The listing builds one solid part. Answer for the finished solid, in the listing's coordinates (mm). A direction names the side the tool comes from. Round coordinates to 2 decimals unless told otherwise and drop trailing zeros. Loops run counter-clockwise (first coordinate to the right, second up) from the corner with the lowest first, then second, coordinate; pieces in that order, holes last. Notation, with made-up numbers: (-12, 72.5) -> (-5, 72.5) arc R19 cw to (-5, 107.5) -> close; hole circle Ø11 at (22.5, -25.75). An arc over 180 degrees is marked (long way). Write each question's results on one line, items separated by ' | '. Start each with the question number.
(1) The part is cut by section B-B (y = 4). Determine the outline of the cut face in (x, z).
(2) The part is cut by section C-C (x = -8.5). Determine the outline of the cut face in (y, z).
(3) Flat-ended cylindrical pins translate along their axes: pin 1 (5 mm diameter, centred on y = 18.5, z = 7.5, fed in from -X); pin 2 (3 mm diameter, centred on y = 26, z = 6.5, fed in from -X); pin 3 (5.5 mm diameter, centred on x = 0, z = 0, fed in from -Y); pin 4 (6 mm diameter, centred on x = -6.5, z = -4, fed in from +Y). Find the tip coordinate at first contact, or state that the pin passes through.
(4) For faces 1 (the face through (-5, 22, 2)), 2 (the face through (0, 37, 0)), 3 (the face through (2.86, 7.89, 0.9)), 4 (the face through (0.62, 2.8, -6.29)), determine the directions among +Z, -Z, +X, -X, +Y, -Y from which every point of the face is accessible in a straight line to the end or side of a thin tool.
(5) The part is cut by section A-A (z = 0). Determine the outline of the cut face in (x, y).
(6) Determine the mould class of faces 5 (the face through (2.1, 0, -2.4)), 6 (the face through (0, 16, 0)), 7 (the face through (-6.29, 2.8, -0.62)), 8 (the face through (9.237, 10.846, 3.83)) for opening direction Z: released by +Z, released by -Z, zero draft, split by the parting line, or undercut.
(7) The part is cut by section D-D (z = -7.25). Determine the outline of the cut face in (x, y), plus the area to 3 significant figures.
(8) Straight lines are drawn through the part: probe 1 along Y at (x, z) = (0, -7); probe 2 along Y at (x, z) = (2.25, 5.5); probe 3 along Z at (x, y) = (-4.5, 4). For each, find the intervals that lie inside material, in ascending order.
```python
from build123d import *

# Parameters (mm, degrees)
SKETCH_1_R          = 10
EXTRUDE_1_DEPTH     = 22
SKETCH_2_R          = 4
EXTRUDE_2_DEPTH     = 15
FILLET_1_R          = 1
CHAMFER_1_SIZE      = 1
SKETCH_4_R          = 3
CUT_EXTRUDE_1_DEPTH = 16
SKETCH_3_R          = 1.35
CUT_EXTRUDE_2_DEPTH = 10
SKETCH_5_R          = 1.35
CUT_EXTRUDE_3_DEPTH = 10


with BuildPart() as part:
    # 草图1 → 凸台-拉伸1 (new body)
    with BuildSketch(Plane(origin=(0, 0, 0), x_dir=(1, 0, 0), z_dir=(0, 1, 0))):
        Circle(SKETCH_1_R)
    extrude(amount=EXTRUDE_1_DEPTH)

    # 草图2 → 凸台-拉伸2 (add)
    with BuildSketch(Plane(origin=(0, 22, 0), x_dir=(1, 0, 0), z_dir=(0, 1, 0))):
        Circle(SKETCH_2_R)
    extrude(amount=EXTRUDE_2_DEPTH)

    # 圆角1
    fillet_1_edges = [part.edges().sort_by_distance(p)[0] for p in [
        (-4, 22, 0),
    ]]
    fillet(fillet_1_edges, radius=FILLET_1_R)

    # 倒角1
    chamfer_1_edges = [part.edges().sort_by_distance(p)[0] for p in [
        (-4, 37, 0),
    ]]
    chamfer(chamfer_1_edges, length=CHAMFER_1_SIZE)

    # 草图4 → 切除-拉伸1 (cut)
    with BuildSketch(Plane.XZ):
        Circle(SKETCH_4_R)
    extrude(amount=-CUT_EXTRUDE_1_DEPTH, mode=Mode.SUBTRACT)

    # 草图3 → 切除-拉伸2 (cut)
    with BuildSketch(Plane.XY):
        with Locations((0, 4)):
            Circle(SKETCH_3_R)
    extrude(amount=-CUT_EXTRUDE_2_DEPTH, mode=Mode.SUBTRACT)

    # 草图5 → 切除-拉伸3 (cut)
    with BuildSketch(Plane(origin=(0, 0, 0), x_dir=(0, 0, -1), z_dir=(1, 0, 0))):
        with Locations((0, 4)):
            Circle(SKETCH_5_R)
    extrude(amount=-CUT_EXTRUDE_3_DEPTH, mode=Mode.SUBTRACT)


solid = part.part
```
Checked values:
1) outline: (-9.91, -1.35) arc R10 ccw to (-1.35, -9.91) -> (-1.35, -2.68) arc R3 cw to (-2.68, -1.35) -> close; (-9.91, 1.35) -> (-2.68, 1.35) arc R3 cw (long way) to (1.35, -2.68) -> (1.35, -9.91) arc R10 ccw (long way) to start
2) outline: (0, -5.27) -> (22, -5.27) -> (22, 5.27) -> (0, 5.27) -> close; hole circle Ø2.7 at (4, 0)
3) pin 1: stops at x = -8.66 | pin 2: passes through | pin 3: stops at y = 16 | pin 4: stops at y = 22.07
4) face 1: +Y | face 2: +Z, -Z, +X, -X, +Y | face 3: -Y | face 4: -Z
5) outline: (-10, 0) -> (-3, 0) -> (-3, 2.65) -> (-10, 2.65) -> close; (-10, 5.35) -> (-3, 5.35) -> (-3, 16) -> (3, 16) -> (3, 0) -> (10, 0) -> (10, 22) -> (5, 22) arc R1 cw to (4, 23) -> (4, 36) -> (3, 37) -> (-3, 37) -> (-4, 36) -> (-4, 23) arc R1 cw to (-5, 22) -> (-10, 22) -> close
6) face 5: zero draft | face 6: undercut | face 7: undercut | face 8: split by the parting line
7) outline: (-6.89, 0) -> (6.89, 0) -> (6.89, 22) -> (-6.89, 22) -> close; hole circle Ø2.7 at (0, 4) | area: 297 mm2
8) probe 1: y = 0 to 2.65, 5.35 to 22 | probe 2: y = 0 to 22 | probe 3: z = -8.93 to -1.35, 1.35 to 8.93
